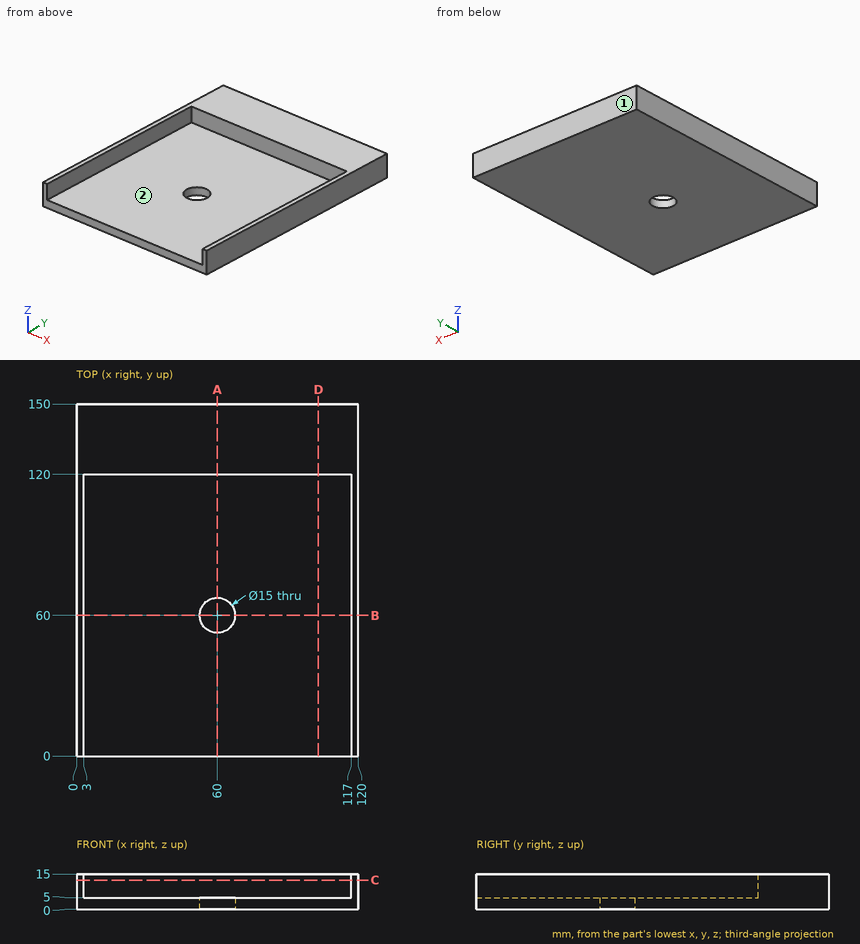
Check sheet for the drawn part. Datum: minimum x, y, z corner. Units: mm. A direction names the side the tool comes from. Round coordinates to 2 decimals unless told otherwise and drop trailing zeros. Loops run counter-clockwise (first coordinate to the right, second up) from the corner with the lowest first, then second, coordinate; pieces in that order, holes last. Notation, with made-up numbers: (31.25, 28.25) - (45.25, 28.25) arc R16 ccw to (45.25, 41.25) - close; hole circle Ø11 at (64, -17). An arc over 180 degrees is marked (long way). Use one line per item in the form item = value.
1. Access from +Z, -Z, +X, -X, +Y, -Y to the whole of each face (thin tool, end or side, straight path). Record for the marked faces 1 and 2.
A:
face_1 = +Z, -Z, +X, -X, +Y
face_2 = +Z, -Y
2. Scan lines: probe 1 along X at (y, z) = (96.5, 11.75); probe 2 along Y at (x, z) = (60, 1.5); probe 3 along Z at (x, y) = (58, 9). Record each from-to range of solid material in increasing order.
A:
probe_1 = 0 to 3, 117 to 120
probe_2 = 0 to 52.5, 67.5 to 150
probe_3 = 0 to 5
3. Section check D-D on x = 103. Record the cut outline in (y, z).
A:
outline = (0, 0) - (150, 0) - (150, 15) - (120, 15) - (120, 5) - (0, 5) - close
4. Gauge pin test, flat ends, axial feed: pin 1 Ø1.5 at (x, y) = (81, 114) entering from +Z; pin 2 Ø5 at (x, z) = (51, 12.5) entering from -Y. Record the tip position at first contact, or that the pin passes through.
A:
pin_1 = 5
pin_2 = 120
5. Section check C-C on z = 12.5. Record the cut outline in (x, y), and give its area (3 significant figures).
A:
outline = (0, 0) - (3, 0) - (3, 120) - (117, 120) - (117, 0) - (120, 0) - (120, 150) - (0, 150) - close
area = 4,320 mm²
6. Section check A-A on x = 60. Record the cut outline in (y, z).
A:
outline = (0, 0) - (52.5, 0) - (52.5, 5) - (0, 5) - close; (67.5, 0) - (150, 0) - (150, 15) - (120, 15) - (120, 5) - (67.5, 5) - close
7. Section check B-B on y = 60. Record the cut outline in (x, z).
A:
outline = (0, 0) - (52.5, 0) - (52.5, 5) - (3, 5) - (3, 15) - (0, 15) - close; (67.5, 0) - (120, 0) - (120, 15) - (117, 15) - (117, 5) - (67.5, 5) - close
